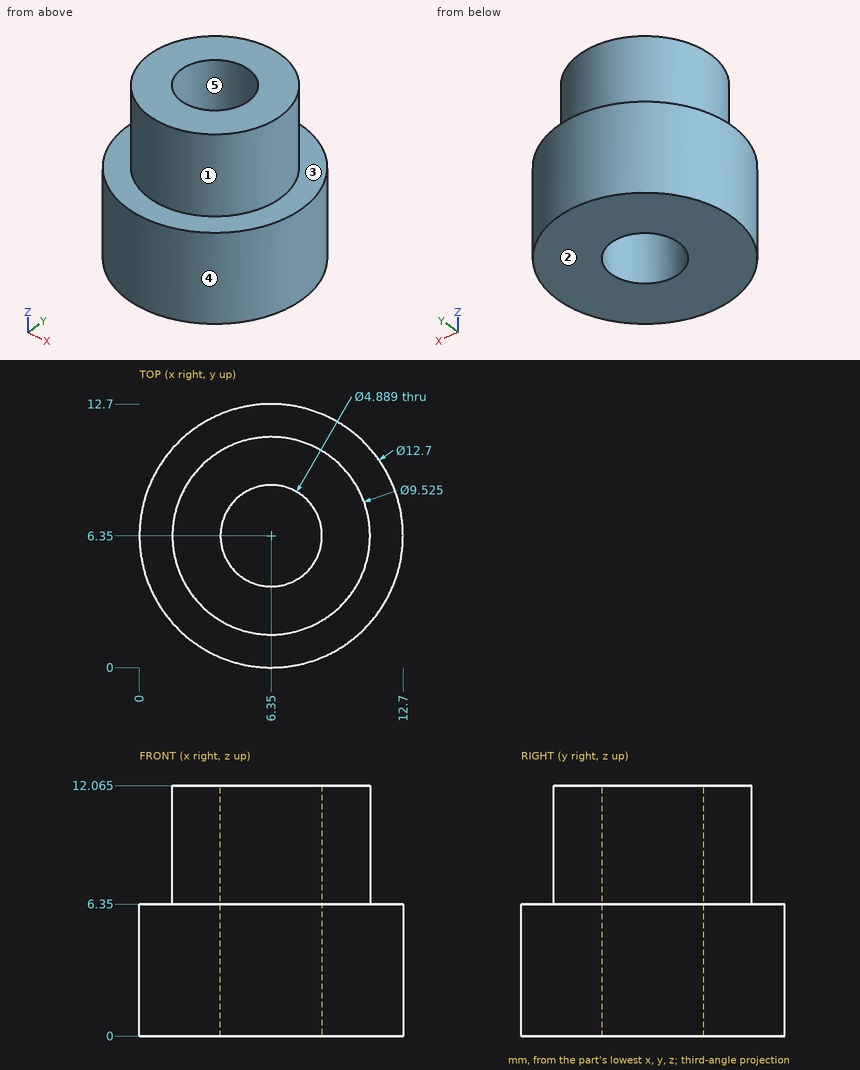
Geometry check sheet. Reference: drawing and pictorial views, mm from the part's lowest x, y, z. A direction names the side the tool comes from. Round coordinates to 2 decimals unless told otherwise and drop trailing zeros. Answer in a Markdown table with one row per item.
(1) Tool access check on the marked faces 1 and 2. Record the directions out of +Z, -Z, +X, -X, +Y, -Y that give a thin tool (end or side, any length) a straight path to the whole face; none if there is none.
Responses:
| item | result |
|---|---|
| face 1 | +Z |
| face 2 | -Z, +X, -X, +Y, -Y |
(2) Draft check along Y on the marked faces 3, 4 and 5. Enter one of: released by +Y, released by -Y, zero draft, split by the parting line, or undercut.
Responses:
| item | result |
|---|---|
| face 3 | zero draft |
| face 4 | split by the parting line |
| face 5 | undercut |
(3) Scan lines: probe 1 along X at (y, z) = (6.5, 7); probe 2 along Z at (x, y) = (10.75, 2.25); probe 3 along X at (y, z) = (6.25, 3). Record each from-to range of solid material in increasing order. Write a range as from..to.
Responses:
| item | result |
|---|---|
| probe 1 | x = 1.59..3.91, 8.79..11.11 |
| probe 2 | z = 0..6.35 |
| probe 3 | x = 0..3.91, 8.79..12.7 |
(4) Go/stop test with flat-tipped pins: P1, Ø2, axis at x = 3.5, y = 11.5, coming from the +Z side; P2, Ø3, axis at y = 7.5, z = 8.5, coming from the -X side; P3, Ø4, axis at x = 2.5, z = 6.5, coming from the +Y side. Record where each tip stops, or that it passes through.
Responses:
| item | result |
|---|---|
| P1 | stops at z = 6.35 |
| P2 | stops at x = 1.59 |
| P3 | stops at y = 12.42 |
